The figure shows three views and two pictorial views of one solid part (mm, origin at its lowest corner). Answer the questions. A direction names the side the tool comes from. Round coordinates to 2 decimals unless told otherwise and drop trailing zeros. Order: outer loops, then holes, each group sorted by start corner. A loop starts at its lowest first (then second) coordinate and runs counter-clockwise, first axis right, second up. Notation, with made-up numbers: (-38, -3) - (-16, -3) arc R19 cw to (-16, 32) - close; hole circle Ø2 at (13.5, 58.25). An arc over 180 degrees is marked (long way). Answer in a Markdown table with one row per item.
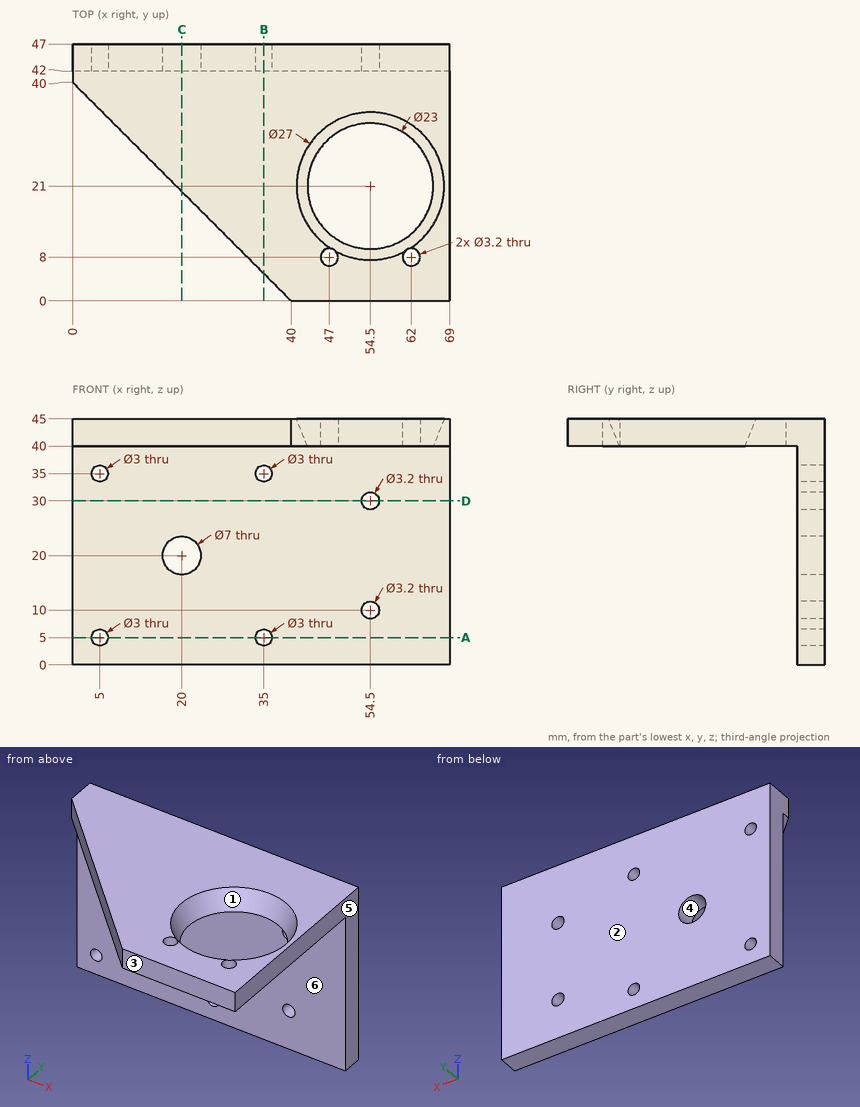
1) Find section D-D, the plane z = 30. Give the vertices of the cut face in (x, y).
Filled in:
| item | result |
|---|---|
| outline | (0, 42) - (52.9, 42) - (52.9, 47) - (0, 47) - close; (56.1, 42) - (69, 42) - (69, 47) - (56.1, 47) - close |
2) Which of the six approach directions +Z, -Z, +X, -X, +Y, -Y give full straight-line access (tool end or side, diameter ignored) to the marked faces 5 and 6?
Filled in:
| item | result |
|---|---|
| face 5 | +Z, -Z, +X, +Y, -Y |
| face 6 | -Z, +X, -X, -Y |
3) Each of these flat-tipped pins is pushed along its axis until it touches: pin 1 (12 mm diameter, centred on x = 19.5, z = 27.5, fed in from -Y); pin 2 (6.5 mm diameter, centred on x = 20, z = 20, fed in from -Y); pin 3 (12 mm diameter, centred on x = 18.5, z = 39, fed in from -Y); pin 4 (1 mm diameter, centred on x = 16.5, y = 30, fed in from -Z). Where does it stop, or does it pass through?
Filled in:
| item | result |
|---|---|
| pin 1 | stops at y = 42 |
| pin 2 | passes through |
| pin 3 | stops at y = 15.58 |
| pin 4 | stops at z = 40 |
4) Find the intervals of material crossed by probe 1 along Z at (x, y) = (54.5, 43.6); probe 2 along Z at (x, y) = (35, 43.5); probe 3 along Y at (x, z) = (62, 43), in increasing order. Write a range as from..to.
Filled in:
| item | result |
|---|---|
| probe 1 | z = 0..8.4, 11.6..28.4, 31.6..45 |
| probe 2 | z = 0..3.5, 6.5..33.5, 36.5..45 |
| probe 3 | y = 0..6.4, 9.6..10.75, 31.25..47 |
5) Find section C-C, the plane x = 20. Give the vertices of the cut face in (y, z).
Filled in:
| item | result |
|---|---|
| outline | (20, 40) - (42, 40) - (42, 23.5) - (47, 23.5) - (47, 45) - (20, 45) - close; (42, 0) - (47, 0) - (47, 16.5) - (42, 16.5) - close |
6) Find section A-A, the plane z = 5. Give the vertices of the cut face in (x, y).
Filled in:
| item | result |
|---|---|
| outline | (0, 42) - (3.5, 42) - (3.5, 47) - (0, 47) - close; (6.5, 42) - (33.5, 42) - (33.5, 47) - (6.5, 47) - close; (36.5, 42) - (69, 42) - (69, 47) - (36.5, 47) - close |
7) Find section B-B, the plane x = 35. Give the vertices of the cut face in (y, z), then the cut area to 3 significant figures.
Filled in:
| item | result |
|---|---|
| outline | (5, 40) - (42, 40) - (42, 36.5) - (47, 36.5) - (47, 45) - (5, 45) - close; (42, 0) - (47, 0) - (47, 3.5) - (42, 3.5) - close; (42, 6.5) - (47, 6.5) - (47, 33.5) - (42, 33.5) - close |
| area | 380 mm^2 |
8) The mould has two halves that part along Y. Classify the marked faces 1, 2, 3 and 4: released by +Y, released by -Y, zero draft, split by the parting line, or undercut.
Filled in:
| item | result |
|---|---|
| face 1 | undercut |
| face 2 | released by +Y |
| face 3 | released by -Y |
| face 4 | zero draft |
